from build123d import *

# Parameters (mm, degrees)
SKETCH1_W           = 76.2
SKETCH1_H           = 50.8
BOSS_EXTRUDE1_DEPTH = 3.175
SKETCH2_W           = 50.8
SKETCH2_H           = 53.975
BOSS_EXTRUDE2_DEPTH = 3.175
SKETCH4_R           = 2.286
SKETCH4_R_2         = 8.6995
CUT_EXTRUDE2_DEPTH  = 3.175
SKETCH6_W           = 73.025
SKETCH6_H           = 25.4
CUT_EXTRUDE3_DEPTH  = 3.175


with BuildPart() as part:
    # Sketch1 → Boss-Extrude1 (new body)
    with BuildSketch(Plane(origin=(0, 0, 0), x_dir=(1, 0, 0), z_dir=(0, 1, 0))):
        with Locations((38.1, 25.4)):
            Rectangle(SKETCH1_W, SKETCH1_H)
    extrude(amount=BOSS_EXTRUDE1_DEPTH)

    # Sketch2 → Boss-Extrude2 (add)
    with BuildSketch(Plane.ZY):
        with Locations((-25.4, 26.9875)):
            Rectangle(SKETCH2_W, SKETCH2_H)
    extrude(amount=-BOSS_EXTRUDE2_DEPTH)

    # Sketch4 → Cut-Extrude2 (cut)
    with BuildSketch(Plane(origin=(3.175, 0, 0), x_dir=(0, 0, -1), z_dir=(1, 0, 0))):
        with Locations((10.8966, 28.4988)):
            Circle(SKETCH4_R)
        with Locations((39.9034, 28.4988)):
            Circle(SKETCH4_R)
        with Locations((25.4, 28.4988)):
            Circle(SKETCH4_R_2)
    extrude(amount=-CUT_EXTRUDE2_DEPTH, mode=Mode.SUBTRACT)

    # Sketch6 → Cut-Extrude3 (cut)
    with BuildSketch(Plane(origin=(0, 3.175, 0), x_dir=(1, 0, 0), z_dir=(0, 1, 0))):
        with Locations((39.6875, 12.7)):
            Rectangle(SKETCH6_W, SKETCH6_H)
    extrude(amount=-CUT_EXTRUDE3_DEPTH, mode=Mode.SUBTRACT)


solid = part.part
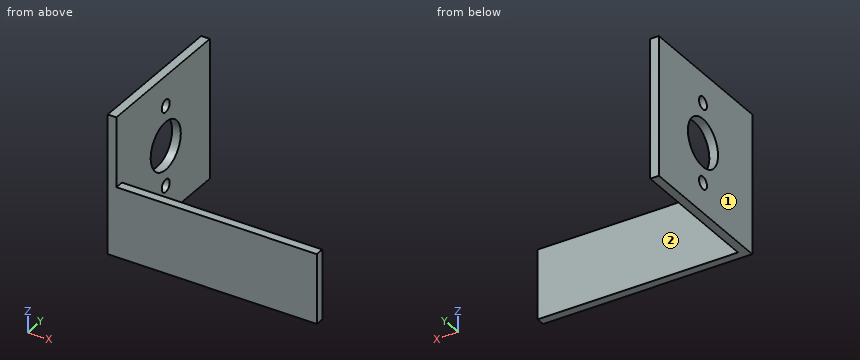
Read the model definition and answer for the solid it produces. Units are mm, in the model's axes. Face numbers are marked on the shaded views. A direction names the side the tool comes from. Round coordinates to 2 decimals unless told otherwise and drop trailing zeros. Write each loop counter-clockwise with the first axis right and the second up, starting at its lowest first coordinate (ties: lowest second). Pieces come first, ordered by that corner, then holes.
Q1. Straight lines are drawn through the part: line 1 (Y direction, x = 1, z = -25) (1 decimal); line 2 (Y direction, x = 8, z = -44) (3 decimals). For each, find the intervals that lie inside material, in ascending order.
Values:
line 1: y = 0 to 19.8, 37.2 to 54
line 2: y = 0 to 3.175
Q2. Find section C-C on z = -45. Determine the outline of the cut face in (x, y) (3 decimals).
Values:
outline: (0, 0) - (76.2, 0) - (76.2, 3.175) - (3.175, 3.175) - (3.175, 53.975) - (0, 53.975) - close
Q3. Find section B-B on y = 47. Determine the outline of the cut face in (x, z) (3 decimals), and give its area (3 significant figures).
Values:
outline: (0, -50.8) - (3.175, -50.8) - (3.175, 0) - (0, 0) - close
area: 161 mm2
Q4. Find section A-A on z = -28. Determine the outline of the cut face in (x, y) (3 decimals).
Values:
outline: (0, 0) - (76.2, 0) - (76.2, 3.175) - (3.175, 3.175) - (3.175, 20.197) - (0, 20.197) - close; (0, 36.801) - (3.175, 36.801) - (3.175, 53.975) - (0, 53.975) - close
Q5. A tool of negligible diameter and unlimited length cuts with its end or side. For the marked faces 1 and 2, from which of +Z, -Z, +X, -X, +Y, -Y can it reach the whole face along a straight path? Write none if from no direction.
Values:
face 1: +Z, -Z, -X, +Y, -Y
face 2: +Z, -Z, +X, +Y
Q6. Flat-ended cylindrical pins translate along their axes: P1, Ø7.5, axis at y = 28.5, z = -10.9, coming from the +X side (3 decimals); P2, Ø7.5, axis at x = 57.5, z = -40, coming from the +Y side (3 decimals); P3, Ø3.5, axis at x = 26, y = 1.5, coming from the +Z side. Find the tip coordinate at first contact, or state that the pin passes through.
Values:
P1: stops at x = 3.175
P2: stops at y = 3.175
P3: stops at z = -25.4
Q7. Find section D-D on x = 27. Determine the outline of the cut face in (y, z) (3 decimals).
Values:
outline: (0, -50.8) - (3.175, -50.8) - (3.175, -25.4) - (0, -25.4) - close
